The listing builds one solid part. Answer for the finished solid, in the listing's coordinates (mm). A direction names the side the tool comes from. Coordinates: 2 decimals unless noted, no trailing zeros. Order: outer loops, then holes, each group sorted by start corner. A loop starts at its lowest first (then second) coordinate and runs counter-clockwise, first axis right, second up. Notation, with made-up numbers: (68, 49) - (100, 49) arc R34 cw to (100, 82) - close; hole circle Ø4 at (7, 83.25). An arc over 180 degrees is marked (long way). Use a Markdown table: item, result. Add a question column.
Item 1: The part is cut by section B-B, the plane z = 9. Give the vertices of the cut face in (x, y) (3 decimals).
Item 2: The part is cut by section A-A, the plane y = -10.5. Give the vertices of the cut face in (x, z).
Item 3: Flat-ended cylindrical pins translate along their axes: P1, Ø15, axis at x = 0, y = 0, coming from the -Z side; P2, Ø5.5, axis at x = 3, y = 0, coming from the +Z side; P3, Ø12, axis at y = -13, z = 13.5, coming from the -X side. Find the tip coordinate at first contact, or state that the pin passes through.
Item 4: Find the intervals of material crossed by line 1 along Y through (x, z) = (0, 14); line 2 along Y through (x, z) = (0, 23) (3 decimals), in increasing order.
Item 5: The mould has two halves that part along Z. Classify faces 1 (the flat face through (-28, 0, 6.35)), 2 (the flat face through (5, 9, 19.05)), 3 (the flat face through (1, 19.05, 0)), 4 (the flat face through (4, 9, -25.4)): released by +Z, released by -Z, zero draft, split by the parting line, or undercut.
Item 6: The part is cut by section C-C, the plane x = 7. Give the vertices of the cut face in (y, z), then the cut area to 3 significant figures.
Item 7: The part is cut by section D-D, the plane y = 0. Give the vertices of the cut face in (x, z) (3 decimals), then the cut area to 3 significant figures.
Item 8: For faces 5 (the flat face through (27, 0, -6.35)), 6 (the flat face through (5, 9, 12.7)), 7 (the cylindrical face through (-7.559, -5.796, 22.181)), 8 (the cylindrical face through (-7.559, -5.796, -16.008)), determine the directions among +Z, -Z, +X, -X, +Y, -Y from which every point of the face is accessible in a straight line to the end or side of a thin tool.
from build123d import *

# Parameters (mm, degrees)
F0_R     = 19.05
F0_R_2   = 9.525
F1_DEPTH = 25.4
F3_START = -6.35
F2_R     = 12.7
F3_DEPTH = 6.35
F5_DEPTH = 6.35


with BuildPart() as f1:
    # F0 (on Top) → F1 (new body, symmetric)
    with BuildSketch(Plane.XY):
        Circle(F0_R)
        Circle(F0_R_2, mode=Mode.SUBTRACT)
    extrude(amount=F1_DEPTH, both=True)

    # F2 (on face) → F3 (cut)
    with BuildSketch(Plane.XY.offset(25.4).offset(F3_START)):
        Circle(F2_R)
    extrude(amount=-F3_DEPTH, mode=Mode.SUBTRACT)

    # F4 (on Top) → F5 (join, symmetric)
    with BuildSketch(Plane.XY):
        Polygon((-38.1, 19.05), (-38.1, 0), (-38.1, -19.05), (38.1, -19.05), (38.1, 0), (38.1, 19.05), align=None)
    extrude(amount=F5_DEPTH, both=True)


solid = f1.part
Solution:
| question | item | result |
|---|---|---|
| 1 | outline | circle Ø38.1 at (0, 0); hole circle Ø19.05 at (0, 0) |
| 2 | outline | (-38.1, -6.35) - (-15.9, -6.35) - (-15.9, -25.4) - (15.9, -25.4) - (15.9, -6.35) - (38.1, -6.35) - (38.1, 6.35) - (15.9, 6.35) - (15.9, 25.4) - (-15.9, 25.4) - (-15.9, 6.35) - (-38.1, 6.35) - close; hole (-7.14, 12.7) - (7.14, 12.7) - (7.14, 19.05) - (-7.14, 19.05) - close |
| 3 | P1 | stops at z = -6.35 |
| 3 | P2 | stops at z = 6.35 |
| 3 | P3 | stops at x = -17.72 |
| 4 | line 1 | y = -19.05 to -12.7, 12.7 to 19.05 |
| 4 | line 2 | y = -19.05 to -9.525, 9.525 to 19.05 |
| 5 | face 1 | released by +Z |
| 5 | face 2 | undercut |
| 5 | face 3 | zero draft |
| 5 | face 4 | released by -Z |
| 6 | outline | (-19.05, -6.35) - (-17.72, -6.35) - (-17.72, -25.4) - (-6.46, -25.4) - (-6.46, -6.35) - (6.46, -6.35) - (6.46, -25.4) - (17.72, -25.4) - (17.72, -6.35) - (19.05, -6.35) - (19.05, 6.35) - (17.72, 6.35) - (17.72, 25.4) - (6.46, 25.4) - (6.46, 19.05) - (10.6, 19.05) - (10.6, 12.7) - (6.46, 12.7) - (6.46, 6.35) - (-6.46, 6.35) - (-6.46, 12.7) - (-10.6, 12.7) - (-10.6, 19.05) - (-6.46, 19.05) - (-6.46, 25.4) - (-17.72, 25.4) - (-17.72, 6.35) - (-19.05, 6.35) - close |
| 6 | area | 1,290 mm2 |
| 7 | outline | (-38.1, -6.35) - (-19.05, -6.35) - (-19.05, -25.4) - (-9.525, -25.4) - (-9.525, -6.35) - (9.525, -6.35) - (9.525, -25.4) - (19.05, -25.4) - (19.05, -6.35) - (38.1, -6.35) - (38.1, 6.35) - (19.05, 6.35) - (19.05, 25.4) - (9.525, 25.4) - (9.525, 19.05) - (12.7, 19.05) - (12.7, 12.7) - (9.525, 12.7) - (9.525, 6.35) - (-9.525, 6.35) - (-9.525, 12.7) - (-12.7, 12.7) - (-12.7, 19.05) - (-9.525, 19.05) - (-9.525, 25.4) - (-19.05, 25.4) - (-19.05, 6.35) - (-38.1, 6.35) - close |
| 7 | area | 1,650 mm2 |
| 8 | face 5 | -Z, +X |
| 8 | face 6 | none |
| 8 | face 7 | +Z |
| 8 | face 8 | -Z |
